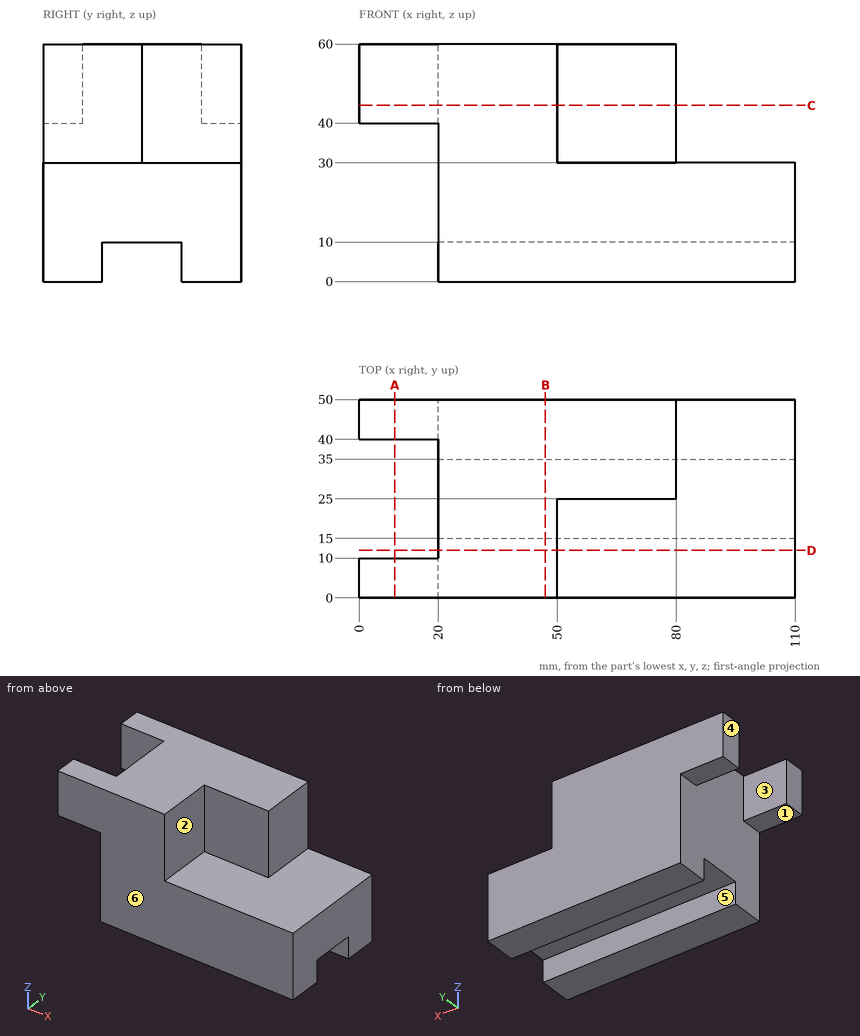
Here's the drawing with two shaded views (mm, measured from the low corner). I have some questions. A direction names the side the tool comes from. Round coordinates to 2 decimals unless told otherwise and drop trailing zeros. Write each loop counter-clockwise with the first axis right and the second up, starting at its lowest first coordinate (ties: lowest second). Pieces come first, ordered by that corner, then holes. Notation, with made-up numbers: M 48.25,72 L 101.25,72 A14 ccw 101.25,86 Z; hole C 52,-21.75 d4. An arc over 180 degrees is marked long. Answer in a Markdown table with one row per item. Add a question column.
Q1. Imagine slicing it at A-A (x = 9). Please give me the cut outline in (y, z), then the cut area to 3 significant figures.
Q2. Imagine slicing it at B-B (x = 47). Please give me the cut outline in (y, z).
Q3. If we mould it in two halves opening along Y, with no side actions, what happens to the marked faces 4, 5 and 6? For each: +Y half, -Y half, draft (parallel to the pull), parting line (faces both ways), or undercut.
Q4. Will these pins go through, and if not, where does the flat tip stop? pin 1 Ø11 at (x, y) = (6.5, 6.5) entering from -Z; pin 2 Ø6 at (x, y) = (49, 25.5) entering from -Z; pin 3 Ø5 at (y, z) = (28, 23.5) entering from -X.
Q5. On a 3-axis mill with a long thin cutter (end or side, diameter ignored), from which of +Z, -Z, +X, -X, +Y, -Y can I reach the whole of each face in a straight line? I mean the marked faces 1, 2 and 3. Say none if no direction works.
Q6. If I drill on line 1 (X direction, y = 32.5, z = 34.5); line 2 (X direction, y = 23, z = 53); line 3 (Y direction, x = 9, z = 43.5), over which ranges is the centre line in solid material (lowest first)? Write a range as from..to.
Q7. Imagine slicing it at D-D (y = 12). Please give me the cut outline in (x, z), then the cut area to 3 significant figures.
Q8. Imagine slicing it at C-C (z = 44.5). Please give me the cut outline in (x, y), then the cut area to 3 significant figures.
Values:
| question | item | result |
|---|---|---|
| 1 | outline | M 0,40 L 10,40 L 10,60 L 0,60 Z; M 40,40 L 50,40 L 50,60 L 40,60 Z |
| 1 | area | 400 mm^2 |
| 2 | outline | M 0,0 L 15,0 L 15,10 L 35,10 L 35,0 L 50,0 L 50,60 L 0,60 Z |
| 3 | face 4 | draft |
| 3 | face 5 | undercut |
| 3 | face 6 | -Y half |
| 4 | pin 1 | z = 40 |
| 4 | pin 2 | z = 10 |
| 4 | pin 3 | x = 20 |
| 5 | face 1 | -Z, -X, +Y, -Y |
| 5 | face 2 | +Z, +X, -Y |
| 5 | face 3 | +Z, -Z, -X |
| 6 | line 1 | 20..80 |
| 6 | line 2 | 20..50 |
| 6 | line 3 | 0..10, 40..50 |
| 7 | outline | M 20,0 L 110,0 L 110,30 L 50,30 L 50,60 L 20,60 Z |
| 7 | area | 3,600 mm^2 |
| 8 | outline | M 0,0 L 50,0 L 50,25 L 80,25 L 80,50 L 0,50 L 0,40 L 20,40 L 20,10 L 0,10 Z |
| 8 | area | 2,650 mm^2 |
